The listing builds one solid part. Answer for the finished solid, in the listing's coordinates (mm). Give positions to 0.01 mm unless a question says otherwise; leave off trailing zeros. Order: outer loops, then holes, each group sorted by start corner. A loop starts at its lowest first (then second) coordinate and runs counter-clockwise, first axis right, second up. Notation, with made-up numbers: (68.25, 39.5) - (122.25, 39.5) arc R36 ccw to (122.25, 73.5) - close; hole circle Ø8 at (-0.5, -1.5). An arc over 180 degrees is marked (long way). Answer as a JSON object with one key per item and string values. Group by question number.
Q1. A cutting plane is placed at A-A, the plane y = 25. Give the vertices of the cut face in (x, z).
Q2. A cutting plane is placed at D-D, the plane y = -4.5. Give the vertices of the cut face in (x, z).
Q3. Given pin 1 (1.5 mm diameter, centred on x = 41, z = 2.5, fed in from -Y); pin 2 (1.5 mm diameter, centred on x = 42.5, z = 2, fed in from +Y); pin 3 (1.5 mm diameter, centred on x = -35, z = 5, fed in from -Y), each flat-ended and moving along its own axis, determine where each tip first touches the part or whether it passes through.
Q4. A cutting plane is placed at B-B, the plane x = -25. Give the vertices of the cut face in (y, z).
Q5. A cutting plane is placed at C-C, the plane z = 2.1. Give the vertices of the cut face in (x, y), and give its area (3 significant figures).
Q6. Consider line 1 (Y direction, x = -39.5, z = 0.7); line 2 (Y direction, x = -25, z = 4.4); line 3 (X direction, y = 9.5, z = 3.9). Determine where each line is inside the solid, lowest interval first.
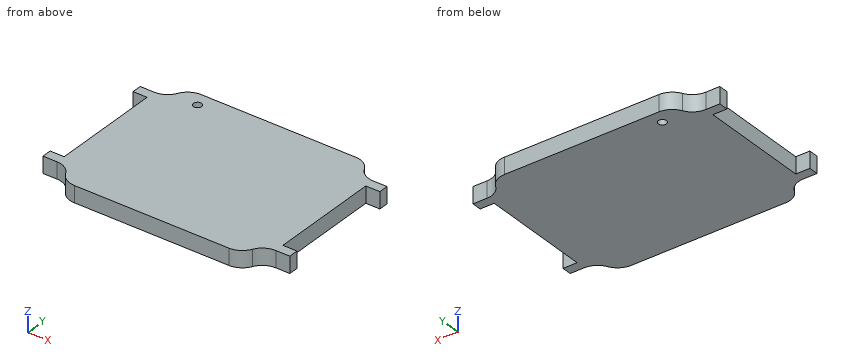
from build123d import *

# Parameters (mm, degrees)
SKETCH1_R           = 1.45
BOSS_EXTRUDE1_DEPTH = 5.85


with BuildPart() as part:
    # Sketch1 → Boss-Extrude1 (new body)
    with BuildSketch(Plane.XY):
        with BuildLine():
            Line((-38.9, 19.6), (-38.9, -19.6))
            Line((-38.9, -19.6), (-43.9, -19.6))
            Line((-43.9, -19.6), (-43.9, -22.98))
            Line((-43.9, -22.98), (-38.9, -22.98))
            ThreePointArc((-38.9, -22.98), (-35.552982671, -23.927877842), (-33.2, -26.49))
            ThreePointArc((-33.2, -26.49), (-30.847017329, -29.052122158), (-27.5, -30))
            Line((-27.5, -30), (27.5, -30))
            ThreePointArc((27.5, -30), (30.847017329, -29.052122158), (33.2, -26.49))
            ThreePointArc((33.2, -26.49), (35.552982671, -23.927877842), (38.9, -22.98))
            Line((38.9, -22.98), (43.9, -22.98))
            Line((43.9, -22.98), (43.9, -19.6))
            Line((43.9, -19.6), (38.9, -19.6))
            Line((38.9, -19.6), (38.9, 19.6))
            Line((38.9, 19.6), (43.9, 19.6))
            Line((43.9, 19.6), (43.9, 22.98))
            Line((43.9, 22.98), (38.9, 22.98))
            ThreePointArc((38.9, 22.98), (35.552982671, 23.927877842), (33.2, 26.49))
            ThreePointArc((33.2, 26.49), (30.847017329, 29.052122158), (27.5, 30))
            Line((27.5, 30), (-27.5, 30))
            ThreePointArc((-27.5, 30), (-30.847017329, 29.052122158), (-33.2, 26.49))
            ThreePointArc((-33.2, 26.49), (-35.552982671, 23.927877842), (-38.9, 22.98))
            Line((-38.9, 22.98), (-43.9, 22.98))
            Line((-43.9, 22.98), (-43.9, 19.6))
            Line((-43.9, 19.6), (-38.9, 19.6))
        make_face()
        with Locations((-25, 25)):
            Circle(SKETCH1_R, mode=Mode.SUBTRACT)
    extrude(amount=BOSS_EXTRUDE1_DEPTH)


solid = part.part
Reply:
{
 "1": {"outline": "(-34.24, 0) - (-26.45, 0) - (-26.45, 5.85) - (-34.24, 5.85) - close; (-23.55, 0) - (34.24, 0) - (34.24, 5.85) - (-23.55, 5.85) - close"},
 "2": {"outline": "(-38.9, 0) - (38.9, 0) - (38.9, 5.85) - (-38.9, 5.85) - close"},
 "3": {"pin 1": "stops at y = -22.98", "pin 2": "stops at y = 22.98", "pin 3": "stops at y = -24.99"},
 "4": {"outline": "(-30, 0) - (23.55, 0) - (23.55, 5.85) - (-30, 5.85) - close; (26.45, 0) - (30, 0) - (30, 5.85) - (26.45, 5.85) - close"},
 "5": {"outline": "(-43.9, -22.98) - (-38.9, -22.98) arc R6.38 cw to (-33.2, -26.49) arc R6.38 ccw to (-27.5, -30) - (27.5, -30) arc R6.38 ccw to (33.2, -26.49) arc R6.38 cw to (38.9, -22.98) - (43.9, -22.98) - (43.9, -19.6) - (38.9, -19.6) - (38.9, 19.6) - (43.9, 19.6) - (43.9, 22.98) - (38.9, 22.98) arc R6.38 cw to (33.2, 26.49) arc R6.38 ccw to (27.5, 30) - (-27.5, 30) arc R6.38 ccw to (-33.2, 26.49) arc R6.38 cw to (-38.9, 22.98) - (-43.9, 22.98) - (-43.9, 19.6) - (-38.9, 19.6) - (-38.9, -19.6) - (-43.9, -19.6) - close; hole circle Ø2.9 at (-25, 25)", "area": "4,570 mm^2"},
 "6": {"line 1": "y = -22.98 to -19.6, 19.6 to 22.98", "line 2": "y = -30 to 23.55, 26.45 to 30", "line 3": "x = -38.9 to 38.9"}
}
